Design review of the part built by this model. Coordinates are the model's own, in mm. Round coordinates to 2 decimals unless told otherwise and drop trailing zeros. Order: outer loops, then holes, each group sorted by start corner. A loop starts at its lowest first (then second) coordinate and runs counter-clockwise, first axis right, second up.
from build123d import *

# Parameters (mm, degrees)
SKETCH1_W               = 40
SKETCH1_H               = 227
BOSS_EXTRUDE1_DEPTH     = 3
SKETCH2_W               = 10
SKETCH2_H               = 3
BOSS_EXTRUDE2_DEPTH     = 3
LPATTERN1_COUNT         = 2
LPATTERN1_PITCH         = 20
SKETCH3_W               = 10
SKETCH3_H               = 3
BOSS_EXTRUDE3_DEPTH     = 3
LPATTERN2_COUNT         = 2
LPATTERN2_PITCH         = 20
SKETCH4_W               = 3
SKETCH4_H               = 10
BOSS_EXTRUDE4_DEPTH     = 3
LPATTERN3_COUNT         = 12
LPATTERN3_PITCH         = 20
ESQUISSE1_W             = 3
ESQUISSE1_H             = 3
ENL_V_MAT_EXTRU_1_DEPTH = 4


with BuildPart() as part:
    # Sketch1 → Boss-Extrude1 (new body)
    with BuildSketch(Plane.XY):
        with Locations((20, 113.5)):
            Rectangle(SKETCH1_W, SKETCH1_H)
    extrude(amount=BOSS_EXTRUDE1_DEPTH)

    # Sketch2 → Boss-Extrude2 (add)
    with BuildSketch(Plane.XZ):
        with Locations((25, 1.5)):
            Rectangle(SKETCH2_W, SKETCH2_H)
    boss_extrude2 = extrude(amount=BOSS_EXTRUDE2_DEPTH)

    # LPattern1: Boss-Extrude2 ×2
    with Locations(*[(-i * LPATTERN1_PITCH, 0, 0) for i in range(1, LPATTERN1_COUNT)]):
        add(boss_extrude2)

    # Sketch3 → Boss-Extrude3 (add)
    with BuildSketch(Plane(origin=(0, 227, 0), x_dir=(1, 0, 0), z_dir=(0, 1, 0))):
        with Locations((25, -1.5)):
            Rectangle(SKETCH3_W, SKETCH3_H)
    boss_extrude3 = extrude(amount=BOSS_EXTRUDE3_DEPTH)

    # LPattern2: Boss-Extrude3 ×2
    with Locations(*[(-i * LPATTERN2_PITCH, 0, 0) for i in range(1, LPATTERN2_COUNT)]):
        add(boss_extrude3)

    # Sketch4 → Boss-Extrude4 (add)
    with BuildSketch(Plane.ZY):
        with Locations((1.5, 5)):
            Rectangle(SKETCH4_W, SKETCH4_H)
    boss_extrude4 = extrude(amount=BOSS_EXTRUDE4_DEPTH)

    # LPattern3: Boss-Extrude4 ×12
    with Locations(*[(0, i * LPATTERN3_PITCH, 0) for i in range(1, LPATTERN3_COUNT)]):
        add(boss_extrude4)

    # Esquisse1 → Enlèv. mat.-Extru.1 (cut, through all)
    with BuildSketch(Plane.XY.offset(3)):
        with Locations((-1.5, 228.5)):
            Rectangle(ESQUISSE1_W, ESQUISSE1_H)
    extrude(amount=-ENL_V_MAT_EXTRU_1_DEPTH, mode=Mode.SUBTRACT)


solid = part.part
1) To check wall thickness, follow line 1 along X through (y, z) = (177, 1.9); line 2 along Y through (x, z) = (12, 2.7). State the ranges of each line that lie inside material, in increasing order.
Results:
line 1: x = 0 to 40
line 2: y = 0 to 227
2) Take a section at A-A on y = 178. Give the boundary of the cut face in (x, z), plus the area to 3 significant figures.
Results:
outline: (0, 0) - (40, 0) - (40, 3) - (0, 3) - close
area: 120 mm2
3) Take a section at B-B on x = 15. Give the boundary of the cut face in (y, z).
Results:
outline: (0, 0) - (227, 0) - (227, 3) - (0, 3) - close
4) Clearance check with flat-ended pins moving along their axes: P1, Ø0.9, axis at x = -1.5, z = 1, coming from the -Y side; P2, Ø0.9, axis at y = -2, z = 1, coming from the -X side; P3, Ø0.9, axis at x = -1, z = 1.5, coming from the +Y side; P4, Ø1, axis at x = 31, y = 125.5, coming from the -Z side. State where each tip first meets the part, or that it passes through.
Results:
P1: stops at y = 0
P2: stops at x = 0
P3: stops at y = 227
P4: stops at z = 0
